Design review of the part built by this model. Coordinates are the model's own, in mm. Face numbers are marked on the shaded views. Round coordinates to 2 decimals unless told otherwise and drop trailing zeros. Loops run counter-clockwise (first coordinate to the right, second up) from the corner with the lowest first, then second, coordinate; pieces in that order, holes last. Notation, with made-up numbers: M 23.5,-20 L 60.5,-20 A9 ccw 60.5,-5 Z; hole C -15,9 d1. An arc over 180 degrees is marked long. Answer as CSV lines item,"result". Start each with the question number.
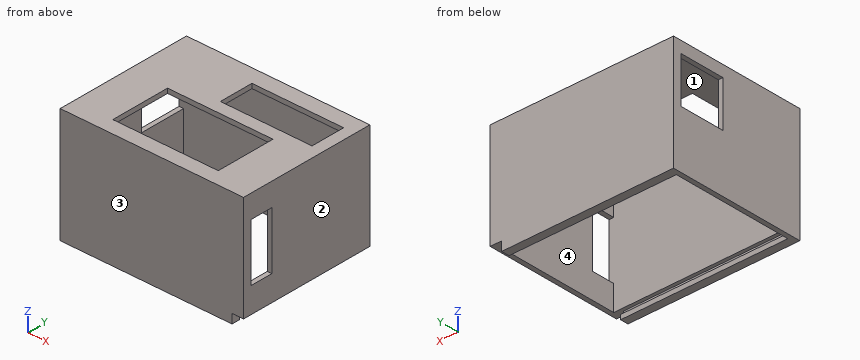
from build123d import *

# Parameters (mm, degrees)
SKETCH_1_W          = 80
SKETCH_1_H          = 60
EXTRUDE_1_DEPTH     = 50
SKETCH_1_3_W        = 76
SKETCH_1_3_H        = 53
CUT_EXTRUDE_1_DEPTH = 48
SKETCH_1_4_W        = 40
SKETCH_1_4_H        = 15
CUT_EXTRUDE_2_DEPTH = 50
SKETCH_1_5_W        = 46
SKETCH_1_5_H        = 26
CUT_EXTRUDE_3_DEPTH = 50
CUT_EXTRUDE_5_DEPTH = 4
CUT_EXTRUDE_START   = 2
SKETCH_1_9_W        = 73
SKETCH_1_9_H        = 56
CUT_EXTRUDE_6_DEPTH = 2
SKETCH_2_W          = 20
SKETCH_2_H          = 20
CUT_EXTRUDE_7_DEPTH = 2
SKETCH_3_W          = 25
SKETCH_3_H          = 10
CUT_EXTRUDE_8_DEPTH = 2


with BuildPart() as part:
    # 草图1 → 凸台-拉伸1 (new body)
    with BuildSketch(Plane.XY):
        with Locations((40, 30)):
            Rectangle(SKETCH_1_W, SKETCH_1_H)
    extrude(amount=EXTRUDE_1_DEPTH)

    # 草图1<3> → 切除-拉伸1 (cut)
    with BuildSketch(Plane.XY):
        with Locations((40, 30)):
            Rectangle(SKETCH_1_3_W, SKETCH_1_3_H)
    extrude(amount=CUT_EXTRUDE_1_DEPTH, mode=Mode.SUBTRACT)

    # 草图1<4> → 切除-拉伸2 (cut)
    with BuildSketch(Plane.XY):
        with Locations((55, 45.5)):
            Rectangle(SKETCH_1_4_W, SKETCH_1_4_H)
    extrude(amount=CUT_EXTRUDE_2_DEPTH, mode=Mode.SUBTRACT)

    # 草图1<5> → 切除-拉伸3 (cut)
    with BuildSketch(Plane.XY):
        with Locations((40, 19.5)):
            Rectangle(SKETCH_1_5_W, SKETCH_1_5_H)
    extrude(amount=CUT_EXTRUDE_3_DEPTH, mode=Mode.SUBTRACT)

    # 草图1<7> → 切除-拉伸5 (cut)
    with BuildSketch(Plane.XY):
        Polygon((75, 2), (75, 0), (80, 0), (80, 60), (75, 60), (75, 58), (75, 56.5), (78, 56.5), (78, 3.5), (75, 3.5), align=None)
    extrude(amount=CUT_EXTRUDE_5_DEPTH, mode=Mode.SUBTRACT)

    # 草图1<9> → 切除-拉伸6 (cut)
    with BuildSketch(Plane.XY.offset(CUT_EXTRUDE_START)):
        with Locations((38.5, 30)):
            Rectangle(SKETCH_1_9_W, SKETCH_1_9_H)
    extrude(amount=CUT_EXTRUDE_6_DEPTH, mode=Mode.SUBTRACT)

    # 草图2 → 切除-拉伸7 (cut)
    with BuildSketch(Plane.ZY):
        with Locations((35, 46.5)):
            Rectangle(SKETCH_2_W, SKETCH_2_H)
    extrude(amount=-CUT_EXTRUDE_7_DEPTH, mode=Mode.SUBTRACT)

    # 草图3 → 切除-拉伸8 (cut)
    with BuildSketch(Plane(origin=(80, 0, 0), x_dir=(0, 0, -1), z_dir=(1, 0, 0))):
        with Locations((-27.5, 8.5)):
            Rectangle(SKETCH_3_W, SKETCH_3_H)
    extrude(amount=-CUT_EXTRUDE_8_DEPTH, mode=Mode.SUBTRACT)


solid = part.part
Item 1: To check wall thickness, follow line 1 (Y direction, x = 76, z = 31.5); line 2 (X direction, y = 40, z = 6); line 3 (Z direction, x = 45.5, y = 57.5). State the ranges of each line that lie inside material, in increasing order.
Item 2: Consider section B-B, the plane y = 49. Write out the cut boundary in (x, z), then the cut area to 3 significant figures.
Item 3: Consider section D-D, the plane x = 74. Write out the cut boundary in (y, z).
Item 4: The part is to be moulded in two halves that separate along X. For the marked faces 1, 2, 3 and 4, say which applies: +X half, -X half, draft (parallel to the pull), parting line (faces both ways), or undercut.
Item 5: Consider section A-A, the plane x = 58.5. Write out the cut boundary in (y, z).
Item 6: Consider section C-C, the plane y = 26.5. Write out the cut boundary in (x, z), then the cut area to 3 significant figures.
Found:
1,line 1,"y = 0 to 3.5, 56.5 to 60"
1,line 2,"x = 0 to 2, 78 to 80"
1,line 3,"z = 0 to 2, 4 to 50"
2,outline,"M 0,0 L 2,0 L 2,25 L 0,25 Z; M 0,45 L 2,45 L 2,48 L 35,48 L 35,50 L 0,50 Z; M 75,48 L 78,48 L 78,4 L 80,4 L 80,50 L 75,50 Z"
2,area,"224 mm^2"
3,outline,"M 0,0 L 3.5,0 L 3.5,2 L 2,2 L 2,4 L 3.5,4 L 3.5,48 L 38,48 L 38,50 L 0,50 Z; M 53,48 L 56.5,48 L 56.5,4 L 58,4 L 58,2 L 56.5,2 L 56.5,0 L 60,0 L 60,50 L 53,50 Z"
4,face 1,"undercut"
4,face 2,"+X half"
4,face 3,"draft"
4,face 4,"undercut"
5,outline,"M 0,0 L 3.5,0 L 3.5,2 L 2,2 L 2,4 L 3.5,4 L 3.5,48 L 6.5,48 L 6.5,50 L 0,50 Z; M 32.5,48 L 38,48 L 38,50 L 32.5,50 Z; M 53,48 L 56.5,48 L 56.5,4 L 58,4 L 58,2 L 56.5,2 L 56.5,0 L 60,0 L 60,50 L 53,50 Z"
6,outline,"M 0,0 L 2,0 L 2,48 L 17,48 L 17,50 L 0,50 Z; M 63,48 L 78,48 L 78,4 L 80,4 L 80,50 L 63,50 Z"
6,area,"252 mm^2"
